Read the model definition and answer for the solid it produces. Units are mm, in the model's axes. A direction names the side the tool comes from. Coordinates: 2 decimals unless noted, no trailing zeros. Write each loop counter-clockwise with the first axis right and the second up, starting at its lowest first coordinate (ties: lowest second). Pieces come first, ordered by that corner, then holes. Notation, with made-up numbers: (28, -21) - (85, -21) arc R19 ccw to (85, -5) - close; hole circle Ø1 at (12.5, -14.75). An arc over 180 degrees is marked (long way). Return JSON: item names as keys, results as strings.
```python
from build123d import *

# Parameters (mm, degrees)
SKETCH_1_R      = 16
EXTRUDE_1_DEPTH = 15
SKETCH_1_3_R    = 45
SKETCH_1_3_R_2  = 16
SKETCH_1_3_R_3  = 12
EXTRUDE_2_DEPTH = 3
SKETCH_1_4_R    = 55
SKETCH_1_4_R_2  = 45
EXTRUDE_3_DEPTH = 11


with BuildPart() as part:
    # Sketch 1 → Extrude 1 (new, symmetric)
    with BuildSketch(Plane.XY):
        Circle(SKETCH_1_R)
        with BuildLine():
            ThreePointArc((-2, 7.228416147), (0, -7.5), (2, 7.228416147))
            Line((2, 7.228416147), (2, 12.022916711))
            Line((2, 12.022916711), (0, 12.022916711))
            Line((0, 12.022916711), (-2, 12.022916711))
            Line((-2, 12.022916711), (-2, 7.228416147))
        make_face(mode=Mode.SUBTRACT)
    extrude(amount=EXTRUDE_1_DEPTH, both=True)

    # Sketch 1_3 → Extrude 2 (add, symmetric)
    with BuildSketch(Plane.XY):
        Circle(SKETCH_1_3_R)
        Circle(SKETCH_1_3_R_2, mode=Mode.SUBTRACT)
        with Locations((16.723776012, 24.906130087)):
            Circle(SKETCH_1_3_R_3, mode=Mode.SUBTRACT)
        with Locations((29.931229371, -2.03014983)):
            Circle(SKETCH_1_3_R_3, mode=Mode.SUBTRACT)
        with Locations((13.207453359, -26.936279917)):
            Circle(SKETCH_1_3_R_3, mode=Mode.SUBTRACT)
        with Locations((-16.723776012, -24.906130087)):
            Circle(SKETCH_1_3_R_3, mode=Mode.SUBTRACT)
        with Locations((-29.931229371, 2.03014983)):
            Circle(SKETCH_1_3_R_3, mode=Mode.SUBTRACT)
        with Locations((-13.207453359, 26.936279917)):
            Circle(SKETCH_1_3_R_3, mode=Mode.SUBTRACT)
    extrude(amount=EXTRUDE_2_DEPTH, both=True)

    # Sketch 1_4 → Extrude 3 (add, symmetric)
    with BuildSketch(Plane.XY):
        Circle(SKETCH_1_4_R)
        Circle(SKETCH_1_4_R_2, mode=Mode.SUBTRACT)
    extrude(amount=EXTRUDE_3_DEPTH, both=True)

    # Sketch 2 → Cut-Revolve 2 (revolve, cut)
    with BuildSketch(Plane(origin=(0, 0, 0), x_dir=(0, 0, -1), z_dir=(1, 0, 0)), mode=Mode.PRIVATE) as cut_revolve_2_sk:
        Polygon((-7.943276133, 55), (-1.5, 55), (-3.221638066, 50), (-6.221638066, 50), align=None)
        Polygon((1.5, 55), (7.943276133, 55), (6.221638066, 50), (3.221638066, 50), align=None)
    revolve(cut_revolve_2_sk.sketch.rotate(Axis((0, 0, 17.503748609), (0, 0, -1)), 90), axis=Axis((0, 0, 17.503748609), (0, 0, -1)), mode=Mode.SUBTRACT)


solid = part.part
```
(1) Flat-ended cylindrical pins translate along their axes: P1, Ø1, axis at x = -6.5, z = 8.5, coming from the -Y side; P2, Ø6, axis at x = -16, z = 7, coming from the -Y side; P3, Ø12, axis at x = 9.5, y = -22, coming from the +Z side; P4, Ø21.5, axis at x = -13.21, y = 26.94, coming from the -Z side. Find the tip coordinate at first contact, or state that the pin passes through.
Answer:
{"P1": "y = -54.67", "P2": "y = -53.4", "P3": "z = 3", "P4": "through"}
(2) Which of the six approach directions +Z, -Z, +X, -X, +Y, -Y give full straight-line access (tool end or side, diameter ignored) to faces 5 (the face through (23.184, 44.574, -6.305)), 6 (the face through (-1, -19, -3)), 7 (the face through (3.33, -6.89, 15)), 8 (the face through (-11.923, -53.692, 0.021)), 9 (the face through (-1, -19, 3))?
Answer:
{"face 5": "none", "face 6": "-Z", "face 7": "+Z, +X, -X, +Y, -Y", "face 8": "+Z, -Z", "face 9": "+Z"}
(3) Straight lines are drawn through the part: line 1 (Z direction, x = -30.5, y = -41); line 2 (Z direction, x = 23, y = -45.5); line 3 (Z direction, x = 44, y = 14.5). For each, find the intervals that lie inside material, in ascending order. Write a range as from..to.
Answer:
{"line 1": "-11..-6.6, -2.84..2.84, 6.6..11", "line 2": "-11..-6.56, -2.88..2.88, 6.56..11", "line 3": "-11..11"}
(4) Determine the mould class of faces 1 (the face through (3.33, -6.89, -15)), 2 (the face through (41.016, -6.626, -0.042)), 3 (the face through (-3.47, -15.62, -8.92)), 4 (the face through (23.22, 44.64, 6.33)) for opening direction Y: +Y half, -Y half, draft (parallel to the pull), parting line (faces both ways), or undercut.
Answer:
{"face 1": "draft", "face 2": "undercut", "face 3": "undercut", "face 4": "parting line"}
(5) A cutting plane is placed at B-B (y = 28.5). State how many separate pieces and enclosed holes the cut face has, and give its area (3 significant figures).
Answer:
{"separate pieces": "3", "enclosed holes": "0", "area": "563 mm²"}
(6) A cutting plane is placed at A-A (z = -4.75). Determine the outline of the cut face in (x, y).
Answer:
{"outline": "circle Ø100 at (0, 0); circle Ø32 at (0, 0); hole circle Ø90 at (0, 0); hole (-2, 7.23) arc R7.5 ccw (long way) to (2, 7.23) - (2, 12.02) - (-2, 12.02) - close"}
